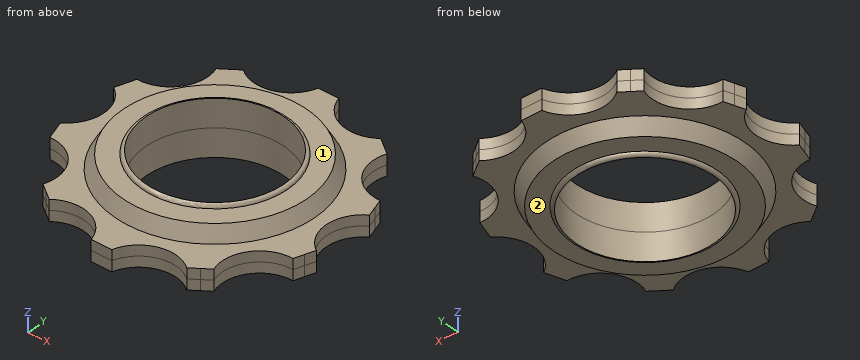
```python
from build123d import *

# Parameters (mm, degrees)
F0_R     = 14.5
F1_DEPTH = 1.5
F0_R_2   = 10.5
F2_DEPTH = 3.5
F0_R_3   = 10
F3_DEPTH = 4
F5_R     = 0.49999


# Not quite as in the source:
# - a fillet or chamfer that OpenCascade refuses, or shapes differently, is made with other operations: its cross-section is extruded or revolved along the edge and cut away or added
# - a fillet or chamfer is up to 0.001 mm smaller than in the source, because OpenCascade refuses the exact size


with BuildPart() as f1:
    # F0 (on Top) → F1 (new body)
    with BuildSketch(Plane.XY):
        with BuildLine():
            Line((-17.7492067955, 7.3442602167), (-18.2127322871, 5.9176754423))
            Line((-18.2127322871, 5.9176754423), (-18.6762577786, 4.4910906678))
            ThreePointArc((-18.6762577786, 4.4910906678), (-16.275, 0), (-18.6762577786, -4.4910906678))
            Line((-18.6762577786, -4.4910906678), (-18.2127322871, -5.9176754423))
            Line((-18.2127322871, -5.9176754423), (-17.7492067955, -7.3442602167))
            ThreePointArc((-17.7492067955, -7.3442602167), (-13.1667515835, -9.5662049811), (-12.469613073, -14.6109975638))
            Line((-12.469613073, -14.6109975638), (-11.2560875814, -15.4926754423))
            Line((-11.2560875814, -15.4926754423), (-10.0425620898, -16.3743533207))
            ThreePointArc((-10.0425620898, -16.3743533207), (-5.0292515835, -15.4784448027), (-1.5, -19.15))
            Line((-1.5, -19.15), (0, -19.15))
            Line((0, -19.15), (1.5, -19.15))
            ThreePointArc((1.5, -19.15), (5.0292515835, -15.4784448027), (10.0425620898, -16.3743533207))
            Line((10.0425620898, -16.3743533207), (11.2560875814, -15.4926754423))
            Line((11.2560875814, -15.4926754423), (12.469613073, -14.6109975638))
            ThreePointArc((12.469613073, -14.6109975638), (13.1667515835, -9.5662049811), (17.7492067955, -7.3442602167))
            Line((17.7492067955, -7.3442602167), (18.2127322871, -5.9176754423))
            Line((18.2127322871, -5.9176754423), (18.6762577786, -4.4910906678))
            ThreePointArc((18.6762577786, -4.4910906678), (16.275, 0), (18.6762577786, 4.4910906678))
            Line((18.6762577786, 4.4910906678), (18.2127322871, 5.9176754423))
            Line((18.2127322871, 5.9176754423), (17.7492067955, 7.3442602167))
            ThreePointArc((17.7492067955, 7.3442602167), (13.1667515835, 9.5662049811), (12.469613073, 14.6109975638))
            Line((12.469613073, 14.6109975638), (11.2560875814, 15.4926754423))
            Line((11.2560875814, 15.4926754423), (10.0425620898, 16.3743533207))
            ThreePointArc((10.0425620898, 16.3743533207), (5.0292515835, 15.4784448027), (1.5, 19.15))
            Line((1.5, 19.15), (0, 19.15))
            Line((0, 19.15), (-1.5, 19.15))
            ThreePointArc((-1.5, 19.15), (-5.0292515835, 15.4784448027), (-10.0425620898, 16.3743533207))
            Line((-10.0425620898, 16.3743533207), (-11.2560875814, 15.4926754423))
            Line((-11.2560875814, 15.4926754423), (-12.469613073, 14.6109975638))
            ThreePointArc((-12.469613073, 14.6109975638), (-13.1667515835, 9.5662049811), (-17.7492067955, 7.3442602167))
        make_face()
        Circle(F0_R, mode=Mode.SUBTRACT)
    extrude(amount=F1_DEPTH)

    # F0 (on Top) → F2 (join)
    with BuildSketch(Plane.XY):
        Circle(F0_R)
        Circle(F0_R_2, mode=Mode.SUBTRACT)
    extrude(amount=F2_DEPTH)

    # F0 (on Top) → F3 (join)
    with BuildSketch(Plane.XY):
        Circle(F0_R_2)
        Circle(F0_R_3, mode=Mode.SUBTRACT)
    extrude(amount=F3_DEPTH)

    # F4: chamfer of 1.2 x 2.0784609691 on 1 edges, made by hand


with BuildPart() as f4_tool2:
    # F4_s3 → F4_t4 (revolve)
    with BuildSketch(Plane.XZ):
        Polygon((14.5, 1.4215390309), (13.3, 3.5), (14.5, 3.5), align=None)
    revolve(axis=Axis((0, 0, 3.5), (0, 0, 1)))

    split(bisect_by=Plane.XY.offset(1.5), keep=Keep.TOP)


with BuildPart() as f1_1:
    add(f1.part)

    # F4_t1: cut F4_tool2
    add(f4_tool2.part, mode=Mode.SUBTRACT)

    # F5 (radius 0.5 in the source; OpenCascade refuses exactly that, so slightly less here)
    f5_edges = [f1_1.edges().sort_by_distance(p)[0] for p in [
        (-10.5, 0, 4),
    ]]
    fillet(f5_edges, radius=F5_R)

    # F6: F1 across face


with BuildPart() as f1_2:
    add(f1_1.part)
    add(f1_1.part.mirror(Plane(origin=(0, 0, 0), x_dir=(1, 0, 0), z_dir=(0, 0, -1))))


solid = f1_2.part
```
Model file for the job. Use its own axes, mm. Face numbers are marked on the shaded views. A direction names the side the tool comes from. Coordinates: 2 decimals unless noted, no trailing zeros. Write each loop counter-clockwise with the first axis right and the second up, starting at its lowest first coordinate (ties: lowest second). Pieces come first, ordered by that corner, then holes. Notation, with made-up numbers: (-16.5, 66) - (9.5, 66) arc R23 ccw to (9.5, 74) - close; hole circle Ø1 at (-34.5, -4). An arc over 180 degrees is marked (long way). One line per item, written item: value. Start each with the question number.
1. Slice it at C-C (z = 1). Write the cut outline in (x, y).
2. Slice it at D-D (x = -15). Write the cut outline in (y, z).
3. Probe line 1 (Y direction, x = 0, z = -0.95); line 2 (X direction, y = 2, z = 1.25); line 3 (X direction, y = 1.5, z = -1.25). List the from-to ranges inside material, lowest first. Write a range as from..to.
4. Flat gauge pin, fed straight in: pin 1 (1.5 mm diameter, centred on x = 8.5, z = -2.5, fed in from -Y). Where does the tip first touch, or does it go through?
5. Tool access for the marked faces 1 and 2: list every direction of +Z, -Z, +X, -X, +Y, -Y with a clear straight run to the whole face (end or side of a thin tool).
Answers below:
1. outline: (-18.68, -4.49) - (-17.75, -7.34) arc R5.4 cw to (-12.47, -14.61) - (-10.04, -16.37) arc R5.4 cw to (-1.5, -19.15) - (1.5, -19.15) arc R5.4 cw to (10.04, -16.37) - (12.47, -14.61) arc R5.4 cw to (17.75, -7.34) - (18.68, -4.49) arc R5.4 cw to (18.68, 4.49) - (17.75, 7.34) arc R5.4 cw to (12.47, 14.61) - (10.04, 16.37) arc R5.4 cw to (1.5, 19.15) - (-1.5, 19.15) arc R5.4 cw to (-10.04, 16.37) - (-12.47, 14.61) arc R5.4 cw to (-17.75, 7.34) - (-18.68, 4.49) arc R5.4 cw to start; hole circle Ø20 at (0, 0)
2. outline: (-7.97, -1.5) - (7.97, -1.5) - (7.97, 1.5) - (-7.97, 1.5) - close
3. line 1: y = -19.15..-10, 10..19.15
3. line 2: x = -16.66..-9.8, 9.8..16.66
3. line 3: x = -16.49..-9.89, 9.89..16.49
4. pin 1: stops at y = -11.73
5. face 1: +Z
5. face 2: -Z
